from build123d import *

# Parameters (mm, degrees)
SKETCH1_R           = 22.098
BOSS_EXTRUDE1_DEPTH = 5.08
SKETCH2_R           = 14.732
BOSS_EXTRUDE2_DEPTH = 35.052
SKETCH3_R           = 11.684
BOSS_EXTRUDE3_DEPTH = 18.796
SKETCH4_R           = 7.747
BOSS_EXTRUDE4_DEPTH = 9.652
SKETCH5_R           = 1.27
BOSS_EXTRUDE5_DEPTH = 7.366
SKETCH6_R           = 1.7907
CUT_EXTRUDE1_DEPTH  = 7.366
CIRPATTERN1_COUNT   = 4
SKETCH7_R           = 12.7
BOSS_EXTRUDE6_DEPTH = 83.82
FILLET1_R           = 5.08


with BuildPart() as part:
    # Sketch1 → Boss-Extrude1 (new body)
    with BuildSketch(Plane(origin=(0, 0, 0), x_dir=(1, 0, 0), z_dir=(0, 1, 0))):
        Circle(SKETCH1_R)
    extrude(amount=BOSS_EXTRUDE1_DEPTH)

    # Sketch2 → Boss-Extrude2 (add)
    with BuildSketch(Plane(origin=(0, 5.08, 0), x_dir=(1, 0, 0), z_dir=(0, 1, 0))):
        Circle(SKETCH2_R)
    extrude(amount=BOSS_EXTRUDE2_DEPTH)

    # Sketch3 → Boss-Extrude3 (add)
    with BuildSketch(Plane(origin=(0, 40.132, 0), x_dir=(1, 0, 0), z_dir=(0, 1, 0))):
        Circle(SKETCH3_R)
    extrude(amount=BOSS_EXTRUDE3_DEPTH)

    # Sketch4 → Boss-Extrude4 (add)
    with BuildSketch(Plane(origin=(0, 58.928, 0), x_dir=(1, 0, 0), z_dir=(0, 1, 0))):
        Circle(SKETCH4_R)
    extrude(amount=BOSS_EXTRUDE4_DEPTH)

    # Sketch5 → Boss-Extrude5 (add)
    with BuildSketch(Plane(origin=(0, 68.58, 0), x_dir=(1, 0, 0), z_dir=(0, 1, 0))):
        with Locations((-4.243406318, 3.044398822)):
            Circle(SKETCH5_R)
        with Locations((2.970026773, -2.481757502)):
            Circle(SKETCH5_R)
    extrude(amount=BOSS_EXTRUDE5_DEPTH)

    # Sketch6 → Cut-Extrude1 (cut)
    with BuildSketch(Plane(origin=(0, 5.08, 0), x_dir=(1, 0, 0), z_dir=(0, 1, 0))):
        with Locations((0, 19.05)):
            Circle(SKETCH6_R)
    cut_extrude1 = extrude(amount=-CUT_EXTRUDE1_DEPTH, mode=Mode.SUBTRACT)

    # CirPattern1: Cut-Extrude1 ×4 about axis
    cirpattern1_axis = Axis((0, 0, 0), (0, 1, 0))
    for i in range(1, CIRPATTERN1_COUNT):
        add(cut_extrude1.rotate(cirpattern1_axis, i * 360 / CIRPATTERN1_COUNT), mode=Mode.SUBTRACT)

    # Sketch7 → Boss-Extrude6 (add)
    with BuildSketch(Plane(origin=(0, 0, 0), x_dir=(-1, 0, 0), z_dir=(0, -1, 0))):
        Circle(SKETCH7_R)
    extrude(amount=BOSS_EXTRUDE6_DEPTH)

    # Fillet1
    fillet1_edges = [part.edges().sort_by_distance(p)[0] for p in [
        (12.7, -83.82, 0),
    ]]
    fillet(fillet1_edges, radius=FILLET1_R)


solid = part.part
Source: CAD feature listing. Evaluate the final solid. Frame: model axes, mm. A direction names the side the tool comes from. Coordinates: 2 decimals unless noted, no trailing zeros. Order: outer loops, then holes, each group sorted by start corner. A loop starts at its lowest first (then second) coordinate and runs counter-clockwise, first axis right, second up. Notation, with made-up numbers: M -1.5,-23 L 15.5,-23 A14 cw 15.5,-6 Z; hole C -37.5,-34.5 d11. An arc over 180 degrees is marked long. Write each question's results on one line, items separated by ' | '. Start each with the question number.
1. Reachability of faces 4 (the face through (4.165, 63.686, -6.532)), 5 (the face through (2.75, -38.82, 12.4)), 6 (the face through (0, -83.82, 0)) from +Z, -Z, +X, -X, +Y, -Y: full face, straight path, thin tool, end or side. Return the list, or none.
2. Draft query along X for faces 1 (the face through (6.8, 22.36, 13.07)), 2 (the face through (-0.233, 2.576, -20.825)), 3 (the face through (4.6, 5.08, 14.4)). Return one class per face: +X half, -X half, draft (parallel to the pull), parting line (faces both ways), or undercut.
3. Pin query (flat end, axial travel): pin 1 (2 mm diameter, centred on y = 16.5, z = -8.5, fed in from +X); pin 2 (4.5 mm diameter, centred on x = 0, z = -19.05, fed in from +Y); pin 3 (4 mm diameter, centred on x = 8, z = -3, fed in from +Y); pin 4 (3 mm diameter, centred on x = 0, z = 19.05, fed in from -Y). Return the tip coordinate at first contact, or that it passes through.
4. Material intervals for L1, parallel to Z at x = 0, y = 2; L2, parallel to Y at x = 10, z = 14, sorted ascending.
5. Section B-B, the plane z = 19.05. Return the cut outline in (x, y).
6. Section C-C, the plane y = 2. Return the cut outline in (x, z).
7. Section D-D, the plane y = -60.5. Return the cut outline in (x, z), then the cut area to 3 significant figures.
8. Section A-A, the plane x = 19.05. Return the cut outline in (y, z), then the cut area to 3 significant figures.
Solution:
1) face 4: +Y | face 5: -Y | face 6: +Z, -Z, +X, -X, -Y
2) face 1: parting line | face 2: undercut | face 3: draft
3) pin 1: x = 12.68 | pin 2: y = 5.08 | pin 3: y = 68.58 | pin 4: through
4) L1: -22.1 to -20.84, -17.26 to 17.26, 20.84 to 22.1 | L2: 0 to 5.08
5) outline: M -11.2,0 L -1.79,0 L -1.79,5.08 L -11.2,5.08 Z; M 1.79,0 L 11.2,0 L 11.2,5.08 L 1.79,5.08 Z
6) outline: C 0,0 d44.2; hole C -19.05,0 d3.58; hole C 0,-19.05 d3.58; hole C 0,19.05 d3.58; hole C 19.05,0 d3.58
7) outline: C 0,0 d25.4 | area: 507 mm²
8) outline: M 0,-11.2 L 5.08,-11.2 L 5.08,-1.79 L 0,-1.79 Z; M 0,1.79 L 5.08,1.79 L 5.08,11.2 L 0,11.2 Z | area: 95.6 mm²
